Part model, mm, in its own coordinate system. A direction names the side the tool comes from. Coordinates: 2 decimals unless noted, no trailing zeros. Loops run counter-clockwise (first coordinate to the right, second up) from the corner with the lowest first, then second, coordinate; pieces in that order, holes last. Notation, with made-up numbers: (-12, 54) - (5, 54) arc R25 cw to (5, 72) - close; hole circle Ø6 at (-26.5, 55). An arc over 180 degrees is marked (long way). Use a Markdown table: item, result. Add a question column.
1) Pull direction Z, two halves, no side cores. Call faces 4 (the face through (90.8, 43.475, 6.468)), 5 (the face through (54, 10.064, 6)), 6 (the face through (105, 6, 9)): +Z half, -Z half, draft (parallel to the pull), parting line (faces both ways), or undercut.
2) Drop flat-ended pins along their axis: P1, Ø6, axis at y = 10, z = 9, coming from the -X side; P2, Ø5, axis at x = 6.5, z = 5, coming from the -Y side; P3, Ø3.5, axis at x = 48.5, z = 7.5, coming from the +Y side; P4, Ø3.5, axis at y = 6.5, z = 5, coming from the -X side. Give the stop position or say it passes through.
3) Band-saw the part on A-A (y = 8.5). Give the cut face in (x, z).
4) Band-saw the part on B-B (x = 52). Give the cut face in (y, z).
5) Tool access for faces 1 (the face through (0, 12, 6)), 2 (the face through (105, 6, 3)), 3 (the face through (4, 14, 8)): list every direction of +Z, -Z, +X, -X, +Y, -Y with a clear straight run to the whole face (end or side of a thin tool).
6) Band-saw the part on C-C (x = 93.5). Give the number of separate pieces and of enclosed holes in the cut face, plus the area to 3 significant figures.
7) Probe probe 1 along X at (y, z) = (41.5, 9.5); probe 2 along Y at (x, z) = (94.5, 2.25); probe 3 along X at (y, z) = (17.5, 7). List the from-to ranges inside material, lowest first. Write a range as [from, to].
from build123d import *

# Parameters (mm, degrees)
ESQUISSE1_W                    = 110
ESQUISSE1_H                    = 14
BOSS_EXTRU_1_DEPTH             = 12
ESQUISSE2_W                    = 6
ESQUISSE2_H                    = 10
ENL_V_MAT_EXTRU_1_DEPTH        = 112.534747949
CONG_1_R                       = 2
ESQUISSE3_W                    = 90
ESQUISSE3_H                    = 10
ENL_V_MAT_EXTRU_2_DEPTH        = 12
CONG_2_R                       = 2
ESQUISSE6_R                    = 4
ESQUISSE6_R_2                  = 2
BOSS_EXTRU_2_DEPTH             = 30
BOSS_EXTRU_2_DIRECTION_2_REACH = 117.782


with BuildPart() as part:
    # Esquisse1 → Boss.-Extru.1 (new body)
    with BuildSketch(Plane.XY):
        with Locations((55, 7)):
            Rectangle(ESQUISSE1_W, ESQUISSE1_H)
    extrude(amount=BOSS_EXTRU_1_DEPTH)

    # Esquisse2 → Enlèv. mat.-Extru.1 (cut, through all)
    with BuildSketch(Plane.ZY):
        with Locations((6, 5)):
            Rectangle(ESQUISSE2_W, ESQUISSE2_H)
    extrude(amount=-ENL_V_MAT_EXTRU_1_DEPTH, mode=Mode.SUBTRACT)

    # Congé1
    # the kernel refuses this fillet: 2 mm, written as the material it takes off along each edge
    with BuildSketch(Plane(origin=(-5, 0, 12), x_dir=(0, 1, 0), z_dir=(1, 0, 0)), Plane(origin=(-5, 0, 9), x_dir=(0, 0, 1), z_dir=(1, 0, 0)), Plane(origin=(-5, 0, 0), x_dir=(0, 0, 1), z_dir=(1, 0, 0))) as cong_1_piece_1:
        with BuildLine():
            CenterArc((CONG_1_R, -CONG_1_R), CONG_1_R, 90, 90)
            Line((0, -CONG_1_R), (0, 0))
            Line((0, 0), (CONG_1_R, 0))
        make_face()
    extrude(amount=120, mode=Mode.SUBTRACT)
    with BuildSketch(Plane(origin=(-5, 0, 3), x_dir=(0, 0, -1), z_dir=(1, 0, 0))) as cong_1_piece_2:
        with BuildLine():
            CenterArc((CONG_1_R, CONG_1_R), CONG_1_R, 180, 90)
            Line((0, CONG_1_R), (0, 0))
            Line((0, 0), (CONG_1_R, 0))
        make_face()
    extrude(amount=120, mode=Mode.SUBTRACT)

    # Esquisse3 → Enlèv. mat.-Extru.2 (cut)
    with BuildSketch(Plane.XY.offset(12)):
        with Locations((55, 5.063508327)):
            Rectangle(ESQUISSE3_W, ESQUISSE3_H)
    extrude(amount=-ENL_V_MAT_EXTRU_2_DEPTH, mode=Mode.SUBTRACT)

    # Congé2
    cong_2_edges = [part.edges().sort_by_distance(p)[0] for p in [
        (55, 10.063508327, 12),
        (55, 10.063508327, 0),
    ]]
    fillet(cong_2_edges, radius=CONG_2_R)

    # Esquisse6 → Boss.-Extru.2 (add)
    # profile 1 of 2: a face of its own
    with BuildSketch(Plane(origin=(-4.499513268, 12.362311102, 0), x_dir=(0, 0, -1), z_dir=(-0.34202014332565694, 0.9396926207859128, 0))):
        with Locations(Location((-8, -8.888282007, 0), (0, 0, 90))):
            Circle(ESQUISSE6_R)
        with Locations(Location((-8, -8.888282007, 0), (0, 0, 90))):
            Circle(ESQUISSE6_R_2, mode=Mode.SUBTRACT)
    # profile 2 of 2: a face of its own
    with BuildSketch(Plane(origin=(-4.499513268, 12.362311102, 0), x_dir=(0, 0, -1), z_dir=(-0.34202014332565694, 0.9396926207859128, 0))):
        with Locations(Location((-8, -103.888282007, 0), (0, 0, 90))):
            Circle(ESQUISSE6_R)
        with Locations(Location((-8, -103.888282007, 0), (0, 0, 90))):
            Circle(ESQUISSE6_R_2, mode=Mode.SUBTRACT)
    extrude(amount=BOSS_EXTRU_2_DEPTH)

    # Esquisse6 → Boss.-Extru.2 direction 2 (add, up to next)
    with BuildSketch(Plane(origin=(-4.499513268, 12.362311102, 0), x_dir=(0, 0, -1), z_dir=(-0.34202014332565694, 0.9396926207859128, 0)), mode=Mode.PRIVATE) as boss_extru_2_direction_2_sk1:
        with Locations(Location((-8, -8.888282007, 0), (0, 0, 90))):
            Circle(ESQUISSE6_R)
        with Locations(Location((-8, -8.888282007, 0), (0, 0, 90))):
            Circle(ESQUISSE6_R_2, mode=Mode.SUBTRACT)
    boss_extru_2_direction_2_tool1 = extrude(boss_extru_2_direction_2_sk1.sketch, amount=-BOSS_EXTRU_2_DIRECTION_2_REACH, mode=Mode.PRIVATE) - part.part
    # Esquisse6 → Boss.-Extru.2 direction 2 (add, up to next)
    with BuildSketch(Plane(origin=(-4.499513268, 12.362311102, 0), x_dir=(0, 0, -1), z_dir=(-0.34202014332565694, 0.9396926207859128, 0)), mode=Mode.PRIVATE) as boss_extru_2_direction_2_sk2:
        with Locations(Location((-8, -103.888282007, 0), (0, 0, 90))):
            Circle(ESQUISSE6_R)
        with Locations(Location((-8, -103.888282007, 0), (0, 0, 90))):
            Circle(ESQUISSE6_R_2, mode=Mode.SUBTRACT)
    boss_extru_2_direction_2_tool2 = extrude(boss_extru_2_direction_2_sk2.sketch, amount=-BOSS_EXTRU_2_DIRECTION_2_REACH, mode=Mode.PRIVATE) - part.part
    add(boss_extru_2_direction_2_tool1.solids().sort_by_distance((7.505196, 16.731668, 8))[0])
    add(boss_extru_2_direction_2_tool2.solids().sort_by_distance((96.775995, 49.223582, 8))[0])


solid = part.part
Answer block:
| question | item | result |
|---|---|---|
| 1 | face 4 | parting line |
| 1 | face 5 | draft |
| 1 | face 6 | undercut |
| 2 | P1 | x = 0 |
| 2 | P2 | y = 0.68 |
| 2 | P3 | y = 14 |
| 2 | P4 | through |
| 3 | outline | (0, 0) - (10, 0) - (10, 3) - (0, 3) - close; (0, 9) - (10, 9) - (10, 12) - (0, 12) - close; (100, 0) - (110, 0) - (110, 3) - (100, 3) - close; (100, 9) - (110, 9) - (110, 12) - (100, 12) - close |
| 4 | outline | (10.06, 2) arc R2 ccw to (12.06, 0) - (14, 0) - (14, 12) - (12.06, 12) arc R2 ccw to (10.06, 10) - close |
| 5 | face 1 | +Z, -Z, -X, -Y |
| 5 | face 2 | +X, -X, -Y |
| 5 | face 3 | none |
| 6 | separate pieces | 2 |
| 6 | enclosed holes | 1 |
| 6 | area | 156 mm2 |
| 7 | probe 1 | [-9.59, -7.05], [-4.24, -1.7], [91.5, 94.04], [96.86, 99.4] |
| 7 | probe 2 | [10.06, 14] |
| 7 | probe 3 | [-1.03, 1.25], [4.93, 7.21], [100.06, 102.34], [106.03, 108.31] |
